```python
from build123d import *

# Parameters (mm, degrees)
SKETCH1_W           = 100
SKETCH1_H           = 100
SKETCH1_R           = 2.2
SKETCH1_R_2         = 1.65
BOSS_EXTRUDE1_DEPTH = 8
SKETCH1_3_R         = 2.15
BOSS_EXTRUDE2_DEPTH = 3
SKETCH1_4_R         = 2.2
CUT_EXTRUDE1_DEPTH  = 4
CHAMFER1_SIZE       = 2


with BuildPart() as part:
    # Sketch1 → Boss-Extrude1 (new body)
    with BuildSketch(Plane(origin=(0, 0, 0), x_dir=(1, 0, 0), z_dir=(0, 1, 0))):
        Rectangle(SKETCH1_W, SKETCH1_H)
        with Locations(Location((40, 40, 0), (0, 0, 270))):
            Circle(SKETCH1_R, mode=Mode.SUBTRACT)
        with Locations(Location((43.713203436, 22.5, 0), (0, 0, 270))):
            Circle(SKETCH1_R_2, mode=Mode.SUBTRACT)
        with Locations(Location((22.5, 43.713203436, 0), (0, 0, 270))):
            Circle(SKETCH1_R_2, mode=Mode.SUBTRACT)
        with Locations(Location((22.5, -43.713203436, 0), (0, 0, 270))):
            Circle(SKETCH1_R_2, mode=Mode.SUBTRACT)
        with Locations(Location((40, -40, 0), (0, 0, 270))):
            Circle(SKETCH1_R, mode=Mode.SUBTRACT)
        with Locations(Location((43.713203436, -22.5, 0), (0, 0, 270))):
            Circle(SKETCH1_R_2, mode=Mode.SUBTRACT)
        with Locations(Location((-43.713203436, -22.5, 0), (0, 0, 270))):
            Circle(SKETCH1_R_2, mode=Mode.SUBTRACT)
        with Locations(Location((-40, -40, 0), (0, 0, 270))):
            Circle(SKETCH1_R, mode=Mode.SUBTRACT)
        with Locations(Location((-22.5, -43.713203436, 0), (0, 0, 270))):
            Circle(SKETCH1_R_2, mode=Mode.SUBTRACT)
        with Locations(Location((-22.5, 43.713203436, 0), (0, 0, 270))):
            Circle(SKETCH1_R_2, mode=Mode.SUBTRACT)
        with Locations(Location((-40, 40, 0), (0, 0, 270))):
            Circle(SKETCH1_R, mode=Mode.SUBTRACT)
        with Locations(Location((-43.713203436, 22.5, 0), (0, 0, 270))):
            Circle(SKETCH1_R_2, mode=Mode.SUBTRACT)
        Polygon((28.7, -27.136195996), (28.7, -22.863804004), (25, -20.727608008), (21.3, -22.863804004), (21.3, -27.136195996), (25, -29.272391992), align=None, mode=Mode.SUBTRACT)
        Polygon((27.136195996, 28.7), (22.863804004, 28.7), (20.727608008, 25), (22.863804004, 21.3), (27.136195996, 21.3), (29.272391992, 25), align=None, mode=Mode.SUBTRACT)
        Polygon((-27.136195996, -28.7), (-22.863804004, -28.7), (-20.727608008, -25), (-22.863804004, -21.3), (-27.136195996, -21.3), (-29.272391992, -25), align=None, mode=Mode.SUBTRACT)
        Polygon((-28.7, 27.136195996), (-28.7, 22.863804004), (-25, 20.727608008), (-21.3, 22.863804004), (-21.3, 27.136195996), (-25, 29.272391992), align=None, mode=Mode.SUBTRACT)
    extrude(amount=BOSS_EXTRUDE1_DEPTH)

    # Sketch1_3 → Boss-Extrude2 (add)
    # profile 1 of 4: a face of its own
    with BuildSketch(Plane(origin=(0, 0, 0), x_dir=(1, 0, 0), z_dir=(0, 1, 0))):
        Polygon((-21.3, 27.136195996), (-25, 29.272391992), (-28.7, 27.136195996), (-28.7, 22.863804004), (-25, 20.727608008), (-21.3, 22.863804004), align=None)
        with Locations(Location((-25, 25, 0), (0, 0, 270))):
            Circle(SKETCH1_3_R, mode=Mode.SUBTRACT)
    # profile 2 of 4: a face of its own
    with BuildSketch(Plane(origin=(0, 0, 0), x_dir=(1, 0, 0), z_dir=(0, 1, 0))):
        Polygon((27.136195996, 21.3), (29.272391992, 25), (27.136195996, 28.7), (22.863804004, 28.7), (20.727608008, 25), (22.863804004, 21.3), align=None)
        with Locations(Location((25, 25, 0), (0, 0, 270))):
            Circle(SKETCH1_3_R, mode=Mode.SUBTRACT)
    # profile 3 of 4: a face of its own
    with BuildSketch(Plane(origin=(0, 0, 0), x_dir=(1, 0, 0), z_dir=(0, 1, 0))):
        Polygon((-27.136195996, -21.3), (-29.272391992, -25), (-27.136195996, -28.7), (-22.863804004, -28.7), (-20.727608008, -25), (-22.863804004, -21.3), align=None)
        with Locations(Location((-25, -25, 0), (0, 0, 270))):
            Circle(SKETCH1_3_R, mode=Mode.SUBTRACT)
    # profile 4 of 4: a face of its own
    with BuildSketch(Plane(origin=(0, 0, 0), x_dir=(1, 0, 0), z_dir=(0, 1, 0))):
        Polygon((21.3, -27.136195996), (25, -29.272391992), (28.7, -27.136195996), (28.7, -22.863804004), (25, -20.727608008), (21.3, -22.863804004), align=None)
        with Locations(Location((25, -25, 0), (0, 0, 270))):
            Circle(SKETCH1_3_R, mode=Mode.SUBTRACT)
    extrude(amount=BOSS_EXTRUDE2_DEPTH)

    # Sketch1_4 → Cut-Extrude1 (cut)
    # profile 1 of 4: a face of its own
    with BuildSketch(Plane(origin=(0, 0, 0), x_dir=(1, 0, 0), z_dir=(0, 1, 0))):
        Polygon((-35.727608008, -40), (-37.863804004, -36.3), (-42.136195996, -36.3), (-44.272391992, -40), (-42.136195996, -43.7), (-37.863804004, -43.7), align=None)
        with Locations(Location((-40, -40, 0), (0, 0, 270))):
            Circle(SKETCH1_4_R, mode=Mode.SUBTRACT)
    # profile 2 of 4: a face of its own
    with BuildSketch(Plane(origin=(0, 0, 0), x_dir=(1, 0, 0), z_dir=(0, 1, 0))):
        Polygon((40, -35.727608008), (36.3, -37.863804004), (36.3, -42.136195996), (40, -44.272391992), (43.7, -42.136195996), (43.7, -37.863804004), align=None)
        with Locations(Location((40, -40, 0), (0, 0, 270))):
            Circle(SKETCH1_4_R, mode=Mode.SUBTRACT)
    # profile 3 of 4: a face of its own
    with BuildSketch(Plane(origin=(0, 0, 0), x_dir=(1, 0, 0), z_dir=(0, 1, 0))):
        Polygon((35.727608008, 40), (37.863804004, 36.3), (42.136195996, 36.3), (44.272391992, 40), (42.136195996, 43.7), (37.863804004, 43.7), align=None)
        with Locations(Location((40, 40, 0), (0, 0, 270))):
            Circle(SKETCH1_4_R, mode=Mode.SUBTRACT)
    # profile 4 of 4: a face of its own
    with BuildSketch(Plane(origin=(0, 0, 0), x_dir=(1, 0, 0), z_dir=(0, 1, 0))):
        Polygon((-40, 35.727608008), (-36.3, 37.863804004), (-36.3, 42.136195996), (-40, 44.272391992), (-43.7, 42.136195996), (-43.7, 37.863804004), align=None)
        with Locations(Location((-40, 40, 0), (0, 0, 270))):
            Circle(SKETCH1_4_R, mode=Mode.SUBTRACT)
    extrude(amount=CUT_EXTRUDE1_DEPTH, mode=Mode.SUBTRACT)

    # Chamfer1
    chamfer1_edges = [part.edges().sort_by_distance(p)[0] for p in [
        (43.713203436, 0, -24.15),
        (22.5, 0, -45.363203436),
        (22.5, 0, 42.063203436),
        (43.713203436, 0, 20.85),
        (-43.713203436, 0, 20.85),
        (-22.5, 0, 42.063203436),
        (-22.5, 0, -45.363203436),
        (-43.713203436, 0, -24.15),
    ]]
    chamfer(chamfer1_edges, length=CHAMFER1_SIZE)


solid = part.part
```
Read the model definition and answer for the solid it produces. Units are mm, in the model's axes. A direction names the side the tool comes from. Round coordinates to 2 decimals unless told otherwise and drop trailing zeros. One line per item, written item: value.
Q1. A flat-ended cylindrical pin translates along its axis: pin 1 Ø8 at (x, z) = (-38.5, -41.5) entering from -Y. Find the tip coordinate at first contact, or state that the pin passes through.
Data:
pin 1: y = 0
Q2. For a pull along Z with two mould halves and no side action, classify faces 1 (the flat face through (50, 4, 1)), 2 (the cylindrical face through (-22.004, 4.958, 45.287)), 3 (the flat face through (-1, 4, 50)) as +Z half, -Z half, draft (parallel to the pull), parting line (faces both ways), or undercut.
Data:
face 1: draft
face 2: undercut
face 3: +Z half
Q3. Which of the six approach directions +Z, -Z, +X, -X, +Y, -Y give full straight-line access (tool end or side, diameter ignored) to faces 4 (the flat face through (21.811, 5.465, -26.876)), 5 (the cylindrical face through (-42.6, 4.96, 21.28)), 6 (the flat face through (42, 4, -42))?
Data:
face 4: +Y
face 5: +Y, -Y
face 6: -Y
Q4. Find section A-A on y = 6. Count the separate pieces of the cut face and the enclosed holes in it, plus the area to 3 significant figures.
Data:
separate pieces: 1
enclosed holes: 16
area: 9,680 mm2
Q5. Straight lines are drawn through the part: line 1 (X direction, y = 6.3, z = -40); line 2 (X direction, y = 3.5, z = -28.5); line 3 (Z direction, x = 23.5, y = 6.75). For each, find the intervals that lie inside material, in ascending order. Write a range as [from, to].
Data:
line 1: [-50, -42.2], [-37.8, 37.8], [42.2, 50]
line 2: [-50, -26.34], [-23.66, 22.75], [27.25, 50]
line 3: [-50, -45.03], [-42.4, -28.7], [-21.3, 21.59], [28.41, 42.4], [45.03, 50]
